Part model, mm, in its own coordinate system. Face numbers are marked on the shaded views. Round coordinates to 2 decimals unless told otherwise and drop trailing zeros. Write each loop counter-clockwise with the first axis right and the second up, starting at its lowest first coordinate (ties: lowest second). Pieces come first, ordered by that corner, then holes. Notation, with made-up numbers: (27.5, 55) -> (61.5, 55) arc R20 ccw to (61.5, 81) -> close; hole circle Ø3 at (-26, 20.25). An arc over 180 degrees is marked (long way). Use CSV: the item, a comma, the result in double quotes. Start each with the question number.
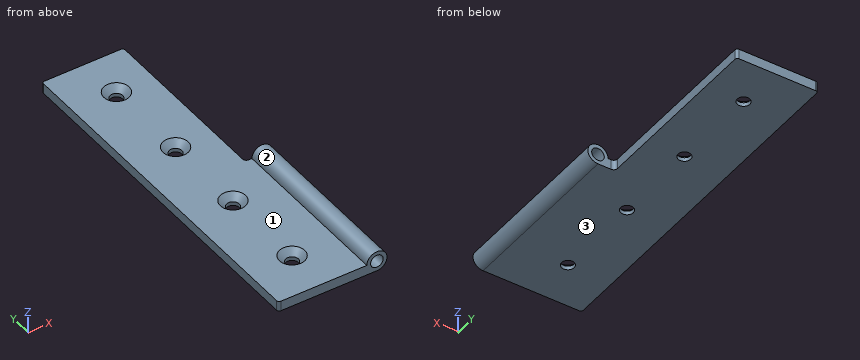
```python
from build123d import *

# Parameters (mm, degrees)
F0_W           = 35
F0_H           = 140
F1_DEPTH       = 4
F2_R           = 2.5
F3_DEPTH       = 68
F6_D           = 5
F6_CSINK_D     = 10
F6_CSINK_ANGLE = 90
F8_DEPTH       = 4.001
F9_R           = 1


with BuildPart() as f1:
    # F0 (on Top) → F1 (new body)
    with BuildSketch(Plane.XY):
        Rectangle(F0_W, F0_H)
    extrude(amount=F1_DEPTH)


with BuildPart() as f3:
    # F2 (on face) → F3 (new body)
    with BuildSketch(Plane.XZ.offset(70)):
        with BuildLine():
            Line((17.5, 4), (17.5, 0))
            Line((17.5, 0), (21.546269994, 0))
            ThreePointArc((21.546269994, 0), (24.3746971188, 6.8284271247), (17.546269994, 4))
            Line((17.546269994, 4), (17.5, 4))
        make_face()
        with Locations((21.546269994, 4)):
            Circle(F2_R, mode=Mode.SUBTRACT)
    extrude(amount=-F3_DEPTH)

    # F4: union F1
    add(f1.part)

    # F6 (through all)
    with Locations(Plane.XY.offset(4)):
        with Locations((0, -52), (0, -17), (0.0200391446, 17), (0, 52)):
            CounterSinkHole(F6_D / 2, F6_CSINK_D / 2, counter_sink_angle=F6_CSINK_ANGLE)

    # F7 (on face) → F8 (cut, through all)
    with BuildSketch(Plane.XY.offset(4)):
        with BuildLine():
            Line((17.5, 70), (14.8238670081, 70))
            Line((14.8238670081, 70), (14.8238670081, -0.5))
            ThreePointArc((14.8238670081, -0.5), (15.2632068363, -1.5606601718), (16.3238670081, -2))
            Line((16.3238670081, -2), (17.5, -2))
            Line((17.5, -2), (17.5, 70))
        make_face()
    extrude(amount=-F8_DEPTH, mode=Mode.SUBTRACT)

    # F9
    f9_edges = [f3.edges().sort_by_distance(p)[0] for p in [
        (-17.5, -70, 2),
        (-17.5, 70, 2),
        (14.823867, 70, 2),
    ]]
    fillet(f9_edges, radius=F9_R)


solid = f3.part
```
1. Band-saw the part on D-D (y = 58.5). List the corners of the cut face in (x, z), then the cut area to 3 significant figures.
2. Band-saw the part on B-B (y = 17). List the corners of the cut face in (x, z).
3. Band-saw the part on C-C (x = -10.5). List the corners of the cut face in (y, z), then the cut area to 3 significant figures.
4. Pull direction Z, two halves, no side cores. Call the marked faces 1, 2 and 3: released by +Z, released by -Z, zero draft, split by the parting line, or undercut.
5. Band-saw the part on A-A (y = -52). List the corners of the cut face in (x, z).
6. Flat gauge pins, fed straight in: pin 1 (6 mm diameter, centred on x = 0, y = 52, fed in from +Z); pin 2 (4 mm diameter, centred on x = -6, z = 7, fed in from +Y); pin 3 (2 mm diameter, centred on y = 31.5, z = 3, fed in from +X); pin 4 (10 mm diameter, centred on x = -2.5, y = 12, fed in from +Z). Where does each tip first touch, or does it go through?
7. Drill centre lines: line 1 along Y through (x, z) = (0, 1.1); line 2 along X through (y, z) = (52, 0.55); line 3 along Z through (x, y) = (8, 13). Where is each one in solid material? Low to high. Write a range as [from, to].
Answers below:
1,outline,"(-17.5, 0) -> (14.82, 0) -> (14.82, 4) -> (-17.5, 4) -> close"
1,area,"129 mm^2"
2,outline,"(-17.5, 0) -> (-2.48, 0) -> (-2.48, 1.5) -> (-4.98, 4) -> (-17.5, 4) -> close; (2.52, 0) -> (14.82, 0) -> (14.82, 4) -> (5.02, 4) -> (2.52, 1.5) -> close"
3,outline,"(-70, 0) -> (70, 0) -> (70, 4) -> (-70, 4) -> close"
3,area,"560 mm^2"
4,face 1,"released by +Z"
4,face 2,"split by the parting line"
4,face 3,"released by -Z"
5,outline,"(-17.5, 0) -> (-2.5, 0) -> (-2.5, 1.5) -> (-5, 4) -> (-17.5, 4) -> close; (2.5, 0) -> (21.55, 0) arc R4 ccw (long way) to (17.55, 4) -> (5, 4) -> (2.5, 1.5) -> close; hole circle Ø5 at (21.55, 4)"
6,pin 1,"stops at z = 2"
6,pin 2,"passes through"
6,pin 3,"stops at x = 14.82"
6,pin 4,"stops at z = 4"
7,line 1,"y = [-70, -54.5], [-49.5, -19.5], [-14.5, 14.5], [19.5, 49.5], [54.5, 70]"
7,line 2,"x = [-17.5, -2.5], [2.5, 14.82]"
7,line 3,"z = [0, 4]"
